from build123d import *

# Parameters (mm, degrees)
F0_W     = 52.832
F0_H     = 32.512
F1_DEPTH = 62.23
F2_T     = -3.81
F3_W     = 5.08
F3_H     = 28.702
F4_DEPTH = 15.24
F6_D     = 4.572
F7_DEPTH = 28.956


with BuildPart() as f1:
    # F0 (on Front) → F1 (new body)
    with BuildSketch(Plane.XZ):
        with Locations((26.416, 16.256)):
            Rectangle(F0_W, F0_H)
    extrude(amount=F1_DEPTH)

    # F2
    f2_openings = [f1.faces().sort_by_distance(p)[0] for p in [
        (26.416, 0, 16.256),
        (26.416, -31.115, 32.512),
        (26.416, -62.23, 16.256),
    ]]
    offset(amount=F2_T, openings=f2_openings)

    # F3 (on face) → F4 (join)
    with BuildSketch(Plane(origin=(49.022, 0, 0), x_dir=(0, -1, 0), z_dir=(-1, 0, 0))):
        with Locations((59.69, 18.161)):
            Rectangle(F3_W, F3_H)
    extrude(amount=F4_DEPTH)

    # F6 (through all)
    with Locations(Plane.XY.offset(3.81)):
        with Locations((12.7508, -4.572), (40.0812, -54.61), (12.7508, -54.61), (40.0812, -4.572)):
            Hole(F6_D / 2)

    # F7 (add): a face of the model
    f7_faces = [f1.faces().sort_by_distance(p)[0] for p in [
        (26.416, -31.1460608146, 0),
    ]]
    extrude(f7_faces, amount=F7_DEPTH)


solid = f1.part
Model file for the job. Use its own axes, mm. A direction names the side the tool comes from. Coordinates: 2 decimals unless noted, no trailing zeros. Write each loop counter-clockwise with the first axis right and the second up, starting at its lowest first coordinate (ties: lowest second). Pieces come first, ordered by that corner, then holes. Notation, with made-up numbers: (45, 50) - (70, 50) arc R23 ccw to (70, 77) - close; hole circle Ø11 at (0, 70). An arc over 180 degrees is marked (long way). Write each question's results on one line, items separated by ' | '. Start each with the question number.
1) Cut at D-D (z = -6.5). Write the cut outline in (x, y), then the cut area to 3 significant figures.
2) 3-axis set-ups, long thin cutter, end or side, ignore diameter. For faces 1 (the face through (33.782, -60, 18)), 2 (the face through (52.832, -31, 2)), 3 (the face through (42, -57.15, 18)): which of +Z, -Z, +X, -X, +Y, -Y reach the whole face in a straight line?
3) Cut at B-B (y = -54.61). Write the cut outline in (x, z), then the cut area to 3 significant figures.
4) Flat gauge pins, fed straight in: P1, Ø6, axis at x = 16.5, y = -36.5, coming from the +Z side; P2, Ø1, axis at x = 10, z = 3, coming from the +Y side; P3, Ø7.5, axis at x = 44.5, z = 17.5, coming from the +Y side. Where does each tip first touch, or does it go through?
5) Cut at C-C (x = 47.5). Write the cut outline in (y, z), then the cut area to 3 significant figures.
6) Cut at A-A (z = 24). Write the cut outline in (x, y).
7) Probe line 1 along X through (y, z) = (-41.5, 8); line 2 along X through (y, z) = (-54, 2); line 3 along Z through (x, y) = (47, -39.5). List the from-to ranges inside material, lowest first. Write a range as from..to.
Returned:
1) outline: (0, -62.23) - (52.83, -62.23) - (52.83, 0) - (0, 0) - close; hole circle Ø4.57 at (12.75, -54.61); hole circle Ø4.57 at (12.75, -4.57); hole circle Ø4.57 at (40.08, -54.61); hole circle Ø4.57 at (40.08, -4.57) | area: 3,220 mm^2
2) face 1: +Z, +Y, -Y | face 2: +Z, -Z, +X, +Y, -Y | face 3: +Z, +Y
3) outline: (0, -28.96) - (10.46, -28.96) - (10.46, 3.81) - (3.81, 3.81) - (3.81, 32.51) - (0, 32.51) - close; (15.04, -28.96) - (37.8, -28.96) - (37.8, 3.81) - (15.04, 3.81) - close; (42.37, -28.96) - (52.83, -28.96) - (52.83, 32.51) - (49.02, 32.51) - (49.02, 3.81) - (42.37, 3.81) - close | area: 1,650 mm^2
4) P1: z = 3.81 | P2: y = 0 | P3: y = -57.15
5) outline: (-62.23, -28.96) - (0, -28.96) - (0, 3.81) - (-57.15, 3.81) - (-57.15, 32.51) - (-62.23, 32.51) - close | area: 2,180 mm^2
6) outline: (0, -62.23) - (3.81, -62.23) - (3.81, 0) - (0, 0) - close; (33.78, -62.23) - (52.83, -62.23) - (52.83, 0) - (49.02, 0) - (49.02, -57.15) - (33.78, -57.15) - close
7) line 1: 0..3.81, 49.02..52.83 | line 2: 0..10.55, 14.95..37.88, 42.28..52.83 | line 3: -28.96..3.81
